Autodesk Inventor part; units mm, degrees
ref_plane "YZ Plane" through (0, 0, 0) normal (1, 0, 0) x (0, 1, 0)
ref_plane "XZ Plane" through (0, 0, 0) normal (0, 1, 0) x (-1, 0, 0)
ref_plane "XY Plane" through (0, 0, 0) normal (0, 0, 1) x (1, 0, 0)
sketch "Sketch1" plane through (0, 0, 0) normal (0, 0, 1) x (1, 0, 0)
  line L0 (0, 0) -> (0, 58.7756)
  line L1 (0, 58.7756) -> (28.6512, 58.7756)
  line L2 (28.6512, 58.7756) -> (28.6512, 0)
  line L3 (28.6512, 0) -> (0, 0)
  line L4 (-9.2202, 67.9958) -> (-9.2202, -9.2202)
  line L5 (-9.2202, -9.2202) -> (37.8714, -9.2202)
  line L6 (37.8714, -9.2202) -> (37.8714, 67.9958)
  line L7 (37.8714, 67.9958) -> (-9.2202, 67.9958)
  dimension "d0" = 28.6512
  dimension "d1" = 58.7756
  dimension "d2" = 9.2202
extrude "Extrusion1" add sketch "Sketch1" along normal blind 10.16
sketch "Sketch2" plane through (0, 0, 10.16) normal (0, 0, 1) x (1, 0, 0)
  line L0 (0, 58.7756) -> (28.6512, 58.7756)
  line L1 (28.6512, 58.7756) -> (28.6512, 0)
  line L2 (28.6512, 0) -> (0, 0)
  line L3 (0, 0) -> (0, 58.7756)
  line L4 (-9.2202, 67.9958) -> (-9.2202, -9.2202)
  line L5 (-9.2202, -9.2202) -> (37.8714, -9.2202)
  line L6 (37.8714, -9.2202) -> (37.8714, 67.9958)
  line L7 (37.8714, 67.9958) -> (-9.2202, 67.9958)
  line L8 (14.3256, 67.9958) -> (14.3256, 58.7756) construction
  line L9 (0, 58.7756) -> (28.6512, 58.7756) construction
  line L10 (14.3256, 63.3857) -> (28.6512, 63.3857) construction
  line L11 (14.3256, 63.3857) -> (0, 63.3857) construction
  circle A0 centre (7.1628, 63.3857) radius 1.7859
  circle A1 centre (21.4884, 63.3857) radius 1.7859
  line L12 (14.3256, 0) -> (14.3256, -9.2202) construction
  line L13 (-9.2202, -9.2202) -> (37.8714, -9.2202) construction
  line L14 (14.3256, -4.6101) -> (0, -4.6101) construction
  line L15 (14.3256, -4.6101) -> (28.6512, -4.6101) construction
  circle A2 centre (7.1628, -4.6101) radius 1.7859
  circle A3 centre (21.4884, -4.6101) radius 1.7859
  dimension "d5" = 3.5719
  dimension "d6" = 3.5719
  dimension "d7" = 3.5719
  dimension "d8" = 3.5719
extrude "Extrusion2" cut sketch "Sketch2" against normal through all contours A0 | A1 | A2 | A3
sketch "Sketch3" plane through (0, 0, 10.16) normal (0, 0, 1) x (1, 0, 0)
  circle A0 centre (7.1628, -4.6101) radius 1.7859
  circle A1 centre (7.1628, 63.3857) radius 1.7859
  circle A2 centre (21.4884, 63.3857) radius 1.7859
  circle A3 centre (21.4884, -4.6101) radius 1.7859
  line L0 (0, 58.7756) -> (28.6512, 58.7756)
  line L1 (28.6512, 58.7756) -> (28.6512, 0)
  line L2 (28.6512, 0) -> (0, 0)
  line L3 (0, 0) -> (0, 58.7756)
  line L4 (-9.2202, 67.9958) -> (-9.2202, -9.2202)
  line L5 (-9.2202, -9.2202) -> (37.8714, -9.2202)
  line L6 (37.8714, -9.2202) -> (37.8714, 67.9958)
  line L7 (37.8714, 67.9958) -> (-9.2202, 67.9958)
  line L8 (-9.2202, 67.9958) -> (-9.2202, -9.2202)
  line L9 (0, 58.7756) -> (-9.2202, 58.7756)
  line L10 (-9.2202, 58.7756) -> (-9.2202, 0)
  line L11 (-9.2202, 0) -> (0, 0)
  line L12 (0, 0) -> (0, 58.7756)
extrude "Extrusion3" cut sketch "Sketch3" against normal through all contours L3 L11 L4 L9
properties part number "New Flipper"
Check sheet for the modelled part. Datum: model origin and axes. Units: mm. A direction names the side the tool comes from. Round coordinates to 2 decimals unless told otherwise and drop trailing zeros. Loops run counter-clockwise (first coordinate to the right, second up) from the corner with the lowest first, then second, coordinate; pieces in that order, holes last. Notation, with made-up numbers: (32.5, 68.25) -> (43.5, 68.25) arc R30 cw to (43.5, 94.25) -> close; hole circle Ø4 at (40, 47.25). An arc over 180 degrees is marked (long way). Write item = value, one per line. Start each with the question number.
1) Sectioned sample at C-C, the plane z = 9. Record the cut outline in (x, y), plus the area to 3 significant figures.
2) Gauge pin test, flat ends, axial feed: pin 1 Ø1 at (y, z) = (47, 7) entering from -X; pin 2 Ø3 at (x, y) = (21.49, -4.61) entering from +Z. Record the tip position at first contact, or that the pin passes through.
3) Sectioned sample at B-B, the plane x = 21. Record the cut outline in (y, z).
4) Set-up check for faces 4 (the flat face through (-9.22, -5, 5)), 5 (the flat face through (9, 0, 5)): record each of +Z, -Z, +X, -X, +Y, -Y from which the full face is reachable in a straight line by a thin tool's end or side.
5) Release check for a two-part mould opening along X. For faces 1 (the cylindrical face through (8.866, -4.074, 5.151)), 2 (the flat face through (28.651, 30, 5)), 3 (the flat face through (15, 67.996, 5)) record: released by +X, released by -X, zero draft, split by the parting line, or undercut.
6) Sectioned sample at A-A, the plane x = 10.5. Record the cut outline in (y, z).
7) Sectioned sample at D-D, the plane y = 32. Record the cut outline in (x, z).
8) Thickness scan on probe 1 along Y at (x, z) = (-4, 9.5); probe 2 along X at (y, z) = (63, 6.5); probe 3 along X at (y, z) = (55.5, 8.25). Record the ranges inside material, lowest first.
Results are:
q1.outline = (-9.22, -9.22) -> (37.87, -9.22) -> (37.87, 68) -> (-9.22, 68) -> (-9.22, 58.78) -> (28.65, 58.78) -> (28.65, 0) -> (-9.22, 0) -> close; hole circle Ø3.57 at (7.16, -4.61); hole circle Ø3.57 at (7.16, 63.39); hole circle Ø3.57 at (21.49, -4.61); hole circle Ø3.57 at (21.49, 63.39)
q1.area = 1,370 mm^2
q2.pin_1 = 28.65
q2.pin_2 = through
q3.outline = (-9.22, 0) -> (-6.33, 0) -> (-6.33, 10.16) -> (-9.22, 10.16) -> close; (-2.89, 0) -> (0, 0) -> (0, 10.16) -> (-2.89, 10.16) -> close; (58.78, 0) -> (61.67, 0) -> (61.67, 10.16) -> (58.78, 10.16) -> close; (65.1, 0) -> (68, 0) -> (68, 10.16) -> (65.1, 10.16) -> close
q4.face_4 = +Z, -Z, -X, +Y, -Y
q4.face_5 = +Z, -Z, -X
q5.face_1 = undercut
q5.face_2 = released by -X
q5.face_3 = zero draft
q6.outline = (-9.22, 0) -> (0, 0) -> (0, 10.16) -> (-9.22, 10.16) -> close; (58.78, 0) -> (68, 0) -> (68, 10.16) -> (58.78, 10.16) -> close
q7.outline = (28.65, 0) -> (37.87, 0) -> (37.87, 10.16) -> (28.65, 10.16) -> close
q8.probe_1 = -9.22 to 0, 58.78 to 68
q8.probe_2 = -9.22 to 5.42, 8.91 to 19.74, 23.23 to 37.87
q8.probe_3 = 28.65 to 37.87
